Part print with two shaded views. Sizes in mm from the minimum x, y, z corner. A direction names the side the tool comes from. Coordinates: 2 decimals unless noted, no trailing zeros. Order: outer loops, then holes, each group sorted by start corner. A loop starts at its lowest first (then second) coordinate and runs counter-clockwise, first axis right, second up. Notation, with made-up numbers: (21, -30) - (29, -30) arc R9 cw to (29, -15) - close; hole circle Ø6 at (30.25, 6.5). An arc over 180 degrees is marked (long way). Return JSON: item names as keys, results as strings.
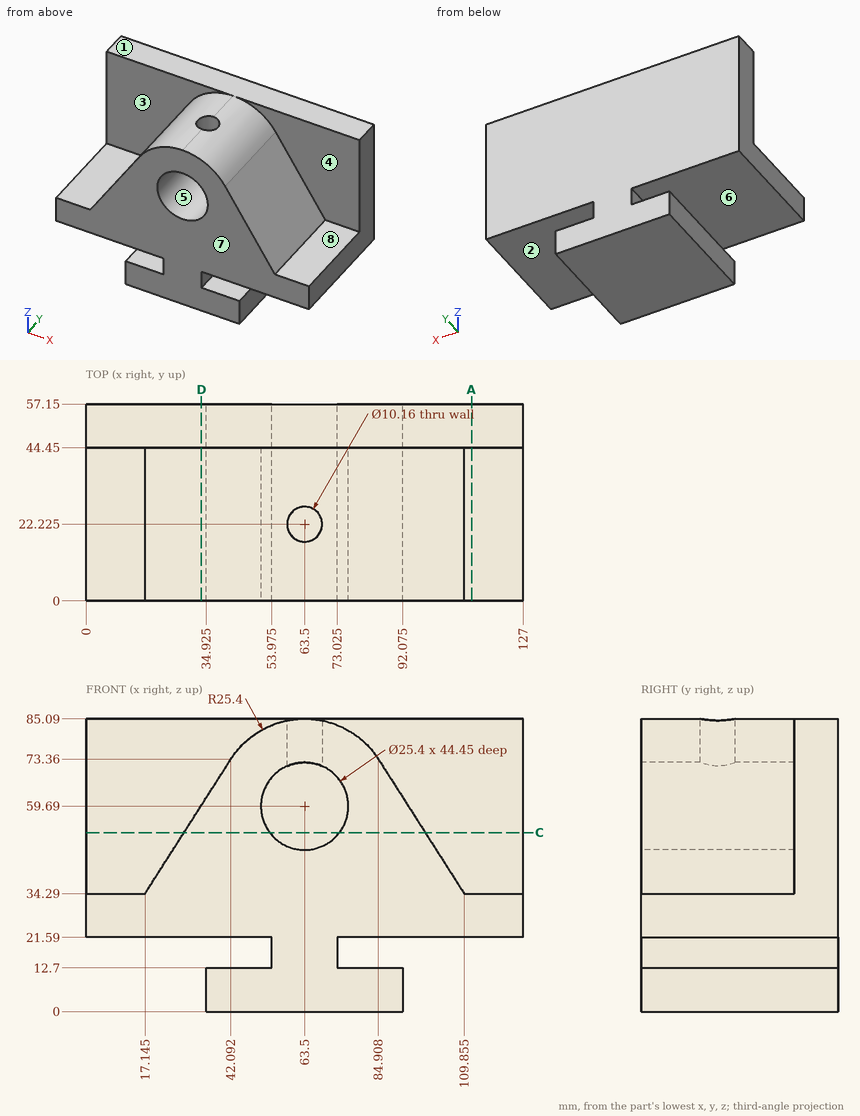
Item 1: Band-saw the part on A-A, the plane x = 112. List the corners of the cut face in (y, z), then the cut area to 3 significant figures.
Findings below:
{"outline": "(0, 21.59) - (57.15, 21.59) - (57.15, 85.09) - (44.45, 85.09) - (44.45, 34.29) - (0, 34.29) - close", "area": "1,370 mm²"}
Item 2: Band-saw the part on D-D, the plane x = 33.5. List the corners of the cut face in (y, z), then the cut area to 3 significant figures.
Findings below:
{"outline": "(0, 21.59) - (57.15, 21.59) - (57.15, 85.09) - (44.45, 85.09) - (44.45, 59.9) - (0, 59.9) - close", "area": "2,510 mm²"}
Item 3: Drop flat-ended pins along their axis: P1, Ø7, axis at y = 28, z = 15, coming from the -X side (3 decimals); P2, Ø8, axis at x = 110.5, y = 47.5, coming from the -Z side; P3, Ø15, axis at x = 80.5, y = 16.5, coming from the +Z side. Give the stop position or say it passes through.
Findings below:
{"P1": "stops at x = 34.925", "P2": "stops at z = 21.59", "P3": "stops at z = 83.25"}
Item 4: Wall check: L1, parallel to Z at x = 37, y = 48.5; L2, parallel to Y at x = 98, z = 53.5; L3, parallel to Z at x = 9, y = 12.5. Give the ranges that are in metal, low to high. Write a range as [from, to].
Findings below:
{"L1": "z = [0, 12.7], [21.59, 85.09]", "L2": "y = [44.45, 57.15]", "L3": "z = [21.59, 34.29]"}
Item 5: Band-saw the part on C-C, the plane z = 52. List the corners of the cut face in (x, y), then the cut area to 3 significant figures.
Findings below:
{"outline": "(0, 44.45) - (28.45, 44.45) - (28.45, 0) - (53.39, 0) - (53.39, 44.45) - (73.61, 44.45) - (73.61, 0) - (98.55, 0) - (98.55, 44.45) - (127, 44.45) - (127, 57.15) - (0, 57.15) - close", "area": "3,830 mm²"}
Item 6: Mould opens along Z. For the marked faces 5, 6, 7 and 8 say: released by +Z, released by -Z, zero draft, split by the parting line, or undercut.
Findings below:
{"face 5": "undercut", "face 6": "undercut", "face 7": "zero draft", "face 8": "released by +Z"}
Item 7: Which spindle directions (+Z, -Z, +X, -X, +Y, -Y) get a long thin tool onto all of the face, cutting with end or side? Do the marked faces 1, 2, 3 and 4. Say none if no direction does.
Findings below:
{"face 1": "+Z, +X, -X, +Y, -Y", "face 2": "+X, +Y, -Y", "face 3": "+Z, -X, -Y", "face 4": "+Z, +X, -Y"}
